from build123d import *

# Parameters (mm, degrees)
SKETCH_1_R          = 1.25
EXTRUDE_1_DEPTH     = 38
SKETCH_2_R          = 2.1
SKETCH_2_W          = 8.5
SKETCH_2_H          = 8.890130192
CUT_EXTRUDE_1_DEPTH = 19


with BuildPart() as part:
    # 草图1 → 凸台-拉伸1 (new body)
    with BuildSketch(Plane(origin=(0, 0, 0), x_dir=(0, 0, -1), z_dir=(1, 0, 0))):
        with BuildLine():
            Line((0, -2.15), (-15, -2.15))
            Line((-15, -2.15), (-15, -1.25))
            Line((-15, -1.25), (-1.749285568, -1.25))
            ThreePointArc((-1.749285568, -1.25), (0.983615779, 1.911805429), (0, -2.15))
        make_face()
        Circle(SKETCH_1_R, mode=Mode.SUBTRACT)
    extrude(amount=EXTRUDE_1_DEPTH)

    # 草图2 → 切除-拉伸1 (cut, symmetric)
    with BuildSketch(Plane(origin=(0, 0, 0), x_dir=(1, 0, 0), z_dir=(0, 1, 0))):
        with Locations((33, -8.5)):
            Circle(SKETCH_2_R)
        with Locations((5, -8.5)):
            Circle(SKETCH_2_R)
        with Locations((33.75, 1.445065096)):
            Rectangle(SKETCH_2_W, SKETCH_2_H)
        with Locations((4.25, 1.445065096)):
            Rectangle(SKETCH_2_W, SKETCH_2_H)
    extrude(amount=CUT_EXTRUDE_1_DEPTH, both=True, mode=Mode.SUBTRACT)


solid = part.part
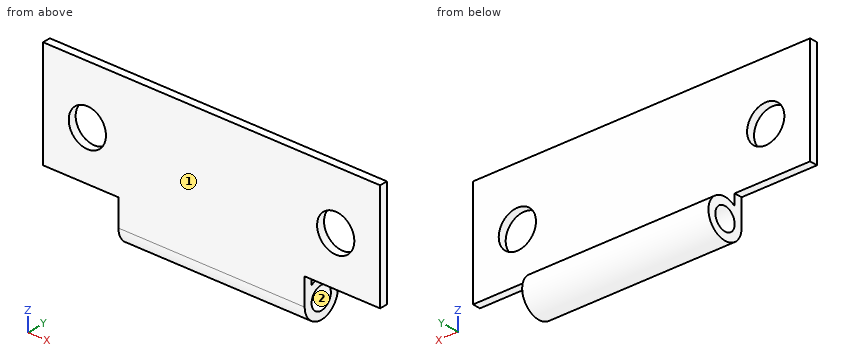
Check sheet for the modelled part. Datum: model origin and axes. Units: mm. Face numbers are marked on the shaded views. Give positions to 0.01 mm unless a question says otherwise; leave off trailing zeros. Write each loop counter-clockwise with the first axis right and the second up, starting at its lowest first coordinate (ties: lowest second). Pieces come first, ordered by that corner, then holes. Notation, with made-up numbers: M 32,-9 L 43,-9 A31 cw 43,21 Z; hole C 56,86 d8. An arc over 180 degrees is marked long. Use one line per item in the form item = value.
(1) Depth check by flat-ended pin: P1, Ø5, axis at x = 33, z = 8.5, coming from the +Y side; P2, Ø2, axis at y = 1, z = 0, coming from the +X side; P3, Ø1.5, axis at y = -1.5, z = -0.5, coming from the -X side. Enter the tip coordinate at first touch or a pass-through.
Answer block:
P1 = -1.25
P2 = 29.5
P3 = 8.5
(2) Material ranges on line 1 along X through (y, z) = (-1.7, 8.5); line 2 along Z through (x, y) = (33, -1.45); line 3 along Y through (x, z) = (26, 9.5), recorded low to high.
Answer block:
line_1 = 0 to 2.9, 7.1 to 30.9, 35.1 to 38
line_2 = 3 to 6.4, 10.6 to 15
line_3 = -2.15 to -1.25
(3) Section check C-C on z = 8.5. Record the boundary of the cut face in (x, y).
Answer block:
outline = M 0,-2.15 L 2.9,-2.15 L 2.9,-1.25 L 0,-1.25 Z; M 7.1,-2.15 L 30.9,-2.15 L 30.9,-1.25 L 7.1,-1.25 Z; M 35.1,-2.15 L 38,-2.15 L 38,-1.25 L 35.1,-1.25 Z
(4) Section check B-B on y = 0. Record the boundary of the cut face in (x, z).
Answer block:
outline = M 8.5,-2.15 L 29.5,-2.15 L 29.5,-1.25 L 8.5,-1.25 Z; M 8.5,1.25 L 29.5,1.25 L 29.5,2.15 L 8.5,2.15 Z
(5) Draft check along Y on the marked faces 1 and 2. Enter one of: pulls with the +Y half, pulls with the -Y half, needs draft (parallel to the pull), parting line crosses it, or undercut.
Answer block:
face_1 = pulls with the -Y half
face_2 = undercut
(6) Section check A-A on x = 33. Record the boundary of the cut face in (y, z), plus the area to 3 significant figures.
Answer block:
outline = M -2.15,3 L -1.25,3 L -1.25,6.4 L -2.15,6.4 Z; M -2.15,10.6 L -1.25,10.6 L -1.25,15 L -2.15,15 Z
area = 7.02 mm2
(7) Section check D-D on y = -1.7. Record the boundary of the cut face in (x, z).
Answer block:
outline = M 0,3 L 8.5,3 L 8.5,-1.32 L 29.5,-1.32 L 29.5,3 L 38,3 L 38,15 L 0,15 Z; hole C 5,8.5 d4.2; hole C 33,8.5 d4.2
